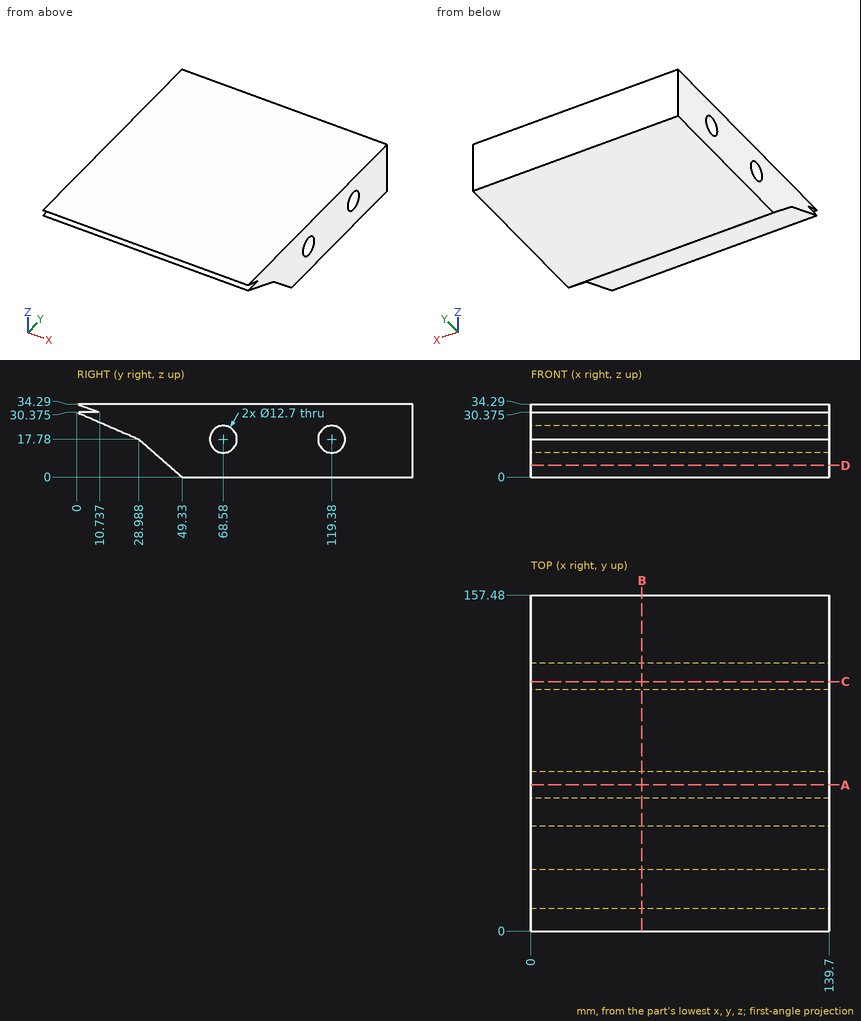
Could you check a few things on this drawing? It's one solid part, dimensions in mm from its lowest x, y, z. Round coordinates to 2 decimals unless told otherwise and drop trailing zeros. Loops run counter-clockwise (first coordinate to the right, second up) from the corner with the lowest first, then second, coordinate; pieces in that order, holes last.
Q1. I want a section at B-B (x = 52). Give the number of separate pieces and of enclosed holes in the cut face, and give its area (3 significant figures).
Q2. I want a section at C-C (y = 117). Write out the boundary of the cut face in (x, z).
Q3. Please list where these lines run through material, in increasing order: L1, parallel to Z at x = 88.5, y = 119.38; L2, parallel to Y at x = 118.5, z = 14 (1 decimal); L3, parallel to Y at x = 56.5, z = 23 (1 decimal).
Q4. I want a section at D-D (z = 5.5). Write out the boundary of the cut face in (x, y).
Q5. I want a section at A-A (y = 68.58). Write out the boundary of the cut face in (x, z), and give its area (3 significant figures).
Q6. For P1, Ø1.5, axis at x = 79.5, z = 8.5, coming from the -Y side, with a flat end and sliding along its axis, tell me the tip position at first contact or that it passes through.
Answer below:
1. separate pieces: 1
1. enclosed holes: 2
1. area: 4,250 mm2
2. outline: (0, 0) - (139.7, 0) - (139.7, 11.89) - (0, 11.89) - close; (0, 23.67) - (139.7, 23.67) - (139.7, 34.29) - (0, 34.29) - close
3. L1: z = 0 to 11.43, 24.13 to 34.29
3. L2: y = 33.3 to 63.5, 73.7 to 114.3, 124.5 to 157.5
3. L3: y = 17 to 65, 72.2 to 115.8, 123 to 157.5
4. outline: (0, 43.04) - (139.7, 43.04) - (139.7, 157.48) - (0, 157.48) - close
5. outline: (0, 0) - (139.7, 0) - (139.7, 11.43) - (0, 11.43) - close; (0, 24.13) - (139.7, 24.13) - (139.7, 34.29) - (0, 34.29) - close
5. area: 3,020 mm2
6. P1: stops at y = 38.75
